```python
from build123d import *

# Parameters (mm, degrees)
F1_DEPTH = 7
F2_SIZE  = 6.99999
F4_DEPTH = 3
F5_SIZE  = 2.99999


# Not quite as in the source:
# - a fillet or chamfer is up to 0.001 mm smaller than in the source, because OpenCascade refuses the exact size


with BuildPart() as f1:
    # F0 (on Front) → F1 (new body)
    with BuildSketch(Plane.XZ):
        Polygon((0, 30), (0, 0), (800, 0), (710, 30), (170, 30), (125, 60), (90, 40), (50, 80), align=None)
        Polygon((800, 0), (0, 0), (0, -30), (50, -80), (90, -40), (125, -60), (170, -30), (710, -30), align=None)
    extrude(amount=F1_DEPTH)

    # F2 (size 7 in the source; OpenCascade refuses exactly that, so slightly less here)
    f2_edges = [f1.edges().sort_by_distance(p)[0] for p in [
        (25, -7, 55),
        (70, -7, 60),
        (107.5, -7, 50),
        (147.5, -7, 45),
        (440, -7, 30),
        (755, -7, 15),
        (25, -7, -55),
        (70, -7, -60),
        (107.5, -7, -50),
        (147.5, -7, -45),
        (440, -7, -30),
        (755, -7, -15),
    ]]
    chamfer(f2_edges, length=F2_SIZE)

    # F3 (on face) → F4 (join)
    with BuildSketch(Plane.XZ.offset(7)):
        Polygon((173.4544423223, -3.2363315113), (190, 0), (0, 0), (0, -16.0339120775), (30.4576978087, -14.7672765888), (60.9153956175, -13.5006411001), (84.8846249282, -11.1722019501), (108.853854239, -8.8437628001), (132.8813694417, -7.6582129113), (156.9088846445, -6.4726630226), align=None)
        Polygon((173.4544423223, 3.2363315113), (190, 0), (174.6631610562, 9.4158361321), align=None)
        Polygon((0, 0), (190, 0), (173.4544423223, 3.2363315113), (156.9088846445, 6.4726630226), (132.8813694417, 7.6582129113), (108.853854239, 8.8437628001), (84.8846249282, 11.1722019501), (60.9153956175, 13.5006411001), (30.4576978087, 14.7672765888), (0, 16.0339120775), align=None)
        Polygon((174.6631610562, -9.4158361321), (190, 0), (173.4544423223, -3.2363315113), align=None)
        Polygon((173.4544423223, 3.2363315113), (174.6631610562, 9.4158361321), (156.9088846445, 6.4726630226), align=None)
        Polygon((174.6631610562, -9.4158361321), (173.4544423223, -3.2363315113), (156.9088846445, -6.4726630226), align=None)
        Polygon((31.0645442111, 29.359591825), (0, 16.0339120775), (30.4576978087, 14.7672765888), align=None)
        Polygon((30.4576978087, -14.7672765888), (0, -16.0339120775), (31.0645442111, -29.359591825), align=None)
        Polygon((132.8813694417, 7.6582129113), (156.9088846445, 6.4726630226), (133.2047409049, 14.2119757014), align=None)
        Polygon((133.2047409049, -14.2119757014), (156.9088846445, -6.4726630226), (132.8813694417, -7.6582129113), align=None)
        Polygon((60.9153956175, 13.5006411001), (31.0645442111, 29.359591825), (30.4576978087, 14.7672765888), align=None)
        Polygon((30.4576978087, -14.7672765888), (31.0645442111, -29.359591825), (60.9153956175, -13.5006411001), align=None)
        Polygon((132.8813694417, 7.6582129113), (133.2047409049, 14.2119757014), (108.853854239, 8.8437628001), align=None)
        Polygon((108.853854239, -8.8437628001), (133.2047409049, -14.2119757014), (132.8813694417, -7.6582129113), align=None)
        Polygon((85.8007351026, 20.602748951), (60.9153956175, 13.5006411001), (84.8846249282, 11.1722019501), align=None)
        Polygon((84.8846249282, -11.1722019501), (60.9153956175, -13.5006411001), (85.8007351026, -20.602748951), align=None)
        Polygon((84.8846249282, 11.1722019501), (108.853854239, 8.8437628001), (85.8007351026, 20.602748951), align=None)
        Polygon((85.8007351026, -20.602748951), (108.853854239, -8.8437628001), (84.8846249282, -11.1722019501), align=None)
    extrude(amount=F4_DEPTH)

    # F5 (size 3 in the source; OpenCascade refuses exactly that, so slightly less here)
    f5_edges = [f1.edges().sort_by_distance(p)[0] for p in [
        (15.532272, -10, 22.696752),
        (45.98997, -10, 21.430116),
        (73.358065, -10, 17.051695),
        (97.327295, -10, 14.723256),
        (121.029298, -10, 11.527869),
        (145.056813, -10, 10.342319),
        (165.786023, -10, 7.94425),
        (182.331581, -10, 4.707918),
        (182.331581, -10, -4.707918),
        (165.786023, -10, -7.94425),
        (145.056813, -10, -10.342319),
        (121.029298, -10, -11.527869),
        (97.327295, -10, -14.723256),
        (73.358065, -10, -17.051695),
        (45.98997, -10, -21.430116),
        (15.532272, -10, -22.696752),
    ]]
    chamfer(f5_edges, length=F5_SIZE)

    # F6: F1 across plane


with BuildPart() as f1_1:
    add(f1.part)
    add(f1.part.mirror(Plane.XZ))


solid = f1_1.part
```
Check sheet for the modelled part. Datum: model origin and axes. Units: mm. A direction names the side the tool comes from. Round coordinates to 2 decimals unless told otherwise and drop trailing zeros. Write each loop counter-clockwise with the first axis right and the second up, starting at its lowest first coordinate (ties: lowest second). Pieces come first, ordered by that corner, then holes. Notation, with made-up numbers: (54.5, 66) -> (92.5, 66) arc R24 ccw to (92.5, 105) -> close; hole circle Ø10 at (74, -39.75). An arc over 180 degrees is marked (long way). One line per question, with ' | ' between items. Start each with the question number.
1. Depth check by flat-ended pin: pin 1 (12 mm diameter, centred on x = 293, y = 2.5, fed in from +Z); pin 2 (2 mm diameter, centred on x = 242, y = 7, fed in from -Z); pin 3 (4 mm diameter, centred on x = 593, y = -7, fed in from +Z). Enter the tip coordinate at first touch or a pass-through.
2. Scan lines: line 1 along Y through (x, z) = (113.5, 42); line 2 along Y through (x, z) = (239.5, -23.5); line 3 along X through (y, z) = (5, 36.5). Record each from-to range of solid material in increasing order. Write a range as from..to.
3. Sectioned sample at A-A, the plane x = 278. Record the cut outline in (y, z), then the cut area to 3 significant figures.
4. Release check for a two-part mould opening along X. For faces 1 (the face through (45.59, 8.52, -19.92)), 2 (the face through (146.74, -3.55, 41.24)), 3 (the face through (24.65, 3.55, -49.63)) record: +X half, -X half, draft (parallel to the pull), parting line (faces both ways), or undercut.
5. Set-up check for faces 4 (the face through (107.2, -3.5, 45.8)), 5 (the face through (97.28, 8.52, 13.04)), 6 (the face through (753.25, 3.55, -11.84)), 7 (the face through (69.07, 3.55, -55.91)), 8 (the face through (69.07, -3.55, -55.91)): record each of +Z, -Z, +X, -X, +Y, -Y from which the full face is reachable in a straight line by a thin tool's end or side.
Taken from the geometry:
1) pin 1: stops at z = 30 | pin 2: stops at z = -24 | pin 3: stops at z = 25
2) line 1: y = -7..7 | line 2: y = -6.5..6.5 | line 3: x = 13.57..86.43, 93.95..151.24
3) outline: (-7, -23) -> (0, -30) -> (7, -23) -> (7, 23) -> (0, 30) -> (-7, 23) -> close | area: 742 mm^2
4) face 1: undercut | face 2: +X half | face 3: -X half
5) face 4: +Z, -Y | face 5: +Z, +Y | face 6: -Z, +X, +Y | face 7: -Z, +Y | face 8: -Z, -Y
